```python
from build123d import *

# Parameters (mm, degrees)
SKETCH1_R                   = 3
BOSS_EXTRUDE1_DEPTH         = 36
TAP_DRILL_FOR_M3_TAP1_D     = 2.5
TAP_DRILL_FOR_M3_TAP1_DEPTH = 10
TAP_DRILL_FOR_M3_TAP1_TIP   = 0.751075774
TAP_DRILL_FOR_M3_TAP2_D     = 2.5
TAP_DRILL_FOR_M3_TAP2_DEPTH = 10
TAP_DRILL_FOR_M3_TAP2_TIP   = 0.751075774


with BuildPart() as part:
    # Sketch1 → Boss-Extrude1 (new body)
    with BuildSketch(Plane(origin=(0, 0, 0), x_dir=(1, 0, 0), z_dir=(0, 1, 0))):
        Circle(SKETCH1_R)
    extrude(amount=BOSS_EXTRUDE1_DEPTH)

    # Tap Drill for M3 Tap1
    with Locations(Plane(origin=(0, 36, 0), x_dir=(1, 0, 0), z_dir=(0, 1, 0))):
        with Locations((0, 0)):
            Hole(TAP_DRILL_FOR_M3_TAP1_D / 2, depth=TAP_DRILL_FOR_M3_TAP1_DEPTH)
            with Locations((0, 0, -(TAP_DRILL_FOR_M3_TAP1_DEPTH + TAP_DRILL_FOR_M3_TAP1_TIP / 2))):  # 118° drill point
                Cone(0, TAP_DRILL_FOR_M3_TAP1_D / 2, TAP_DRILL_FOR_M3_TAP1_TIP, mode=Mode.SUBTRACT)

    # Tap Drill for M3 Tap2
    with Locations(Plane(origin=(0, 0, 0), x_dir=(-1, 0, 0), z_dir=(0, -1, 0))):
        with Locations((0, 0)):
            Hole(TAP_DRILL_FOR_M3_TAP2_D / 2, depth=TAP_DRILL_FOR_M3_TAP2_DEPTH)
            with Locations((0, 0, -(TAP_DRILL_FOR_M3_TAP2_DEPTH + TAP_DRILL_FOR_M3_TAP2_TIP / 2))):  # 118° drill point
                Cone(0, TAP_DRILL_FOR_M3_TAP2_D / 2, TAP_DRILL_FOR_M3_TAP2_TIP, mode=Mode.SUBTRACT)


solid = part.part
```
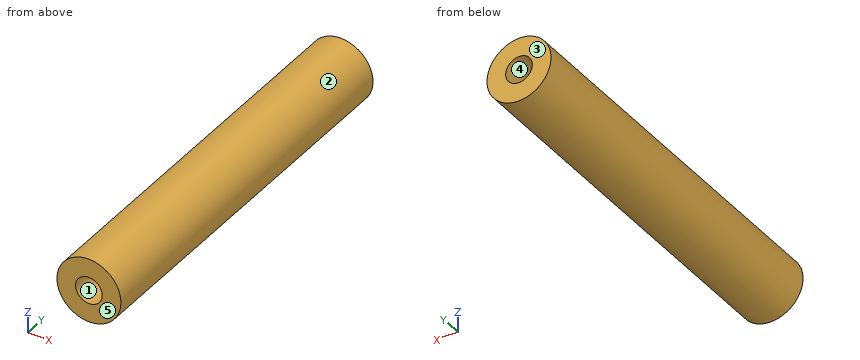
Design review of the part built by this model. Coordinates are the model's own, in mm. Face numbers are marked on the shaded views. A direction names the side the tool comes from. Round coordinates to 2 decimals unless told otherwise and drop trailing zeros. Write each loop counter-clockwise with the first axis right and the second up, starting at its lowest first coordinate (ties: lowest second). Pieces come first, ordered by that corner, then holes. Notation, with made-up numbers: (56, 67) -> (82, 67) arc R8 cw to (82, 73) -> close; hole circle Ø8 at (3.25, 75.25). An arc over 180 degrees is marked (long way). Answer in a Markdown table with one row per item.
Q1. Draft analysis for pull direction Z (two halves, no side actions). For the marked faces 1, 2 and 3, state which applies: +Z half, -Z half, draft (parallel to the pull), parting line (faces both ways), or undercut.
The answers:
| item | result |
|---|---|
| face 1 | undercut |
| face 2 | parting line |
| face 3 | draft |
Q2. Take a section at B-B, the plane z = -2.5. State the section outline as (x, y) points, then the cut area to 3 significant figures.
The answers:
| item | result |
|---|---|
| outline | (-1.66, 0) -> (1.66, 0) -> (1.66, 36) -> (-1.66, 36) -> close |
| area | 119 mm² |
Q3. Take a section at D-D, the plane x = 2.25. State the section outline as (y, z) points, then the cut area to 3 significant figures.
The answers:
| item | result |
|---|---|
| outline | (0, -1.98) -> (36, -1.98) -> (36, 1.98) -> (0, 1.98) -> close |
| area | 143 mm² |
Q4. Take a section at C-C, the plane y = 18. State the section outline as (x, z) points, then the cut area to 3 significant figures.
The answers:
| item | result |
|---|---|
| outline | circle Ø6 at (0, 0) |
| area | 28.3 mm² |
Q5. For the marked faces 4 and 5, list the 3-axis set-ups (+Z, -Z, +X, -X, +Y, -Y) from which the entire face can be reached by the end or side of a thin tool; tool diameter is ignored.
The answers:
| item | result |
|---|---|
| face 4 | +Y |
| face 5 | +Z, -Z, +X, -X, -Y |
Q6. Clearance check with flat-ended pins moving along their axes: pin 1 Ø3 at (y, z) = (9, -0.5) entering from +X; pin 2 Ø2 at (x, z) = (0, 0) entering from -Y; pin 3 Ø1.5 at (x, y) = (-2, 22.5) entering from +Z; pin 4 Ø1.5 at (x, z) = (0, 0) entering from -Y. State where each tip first meets the part, or that it passes through.
The answers:
| item | result |
|---|---|
| pin 1 | x = 3 |
| pin 2 | y = 10.15 |
| pin 3 | z = 2.73 |
| pin 4 | y = 10.3 |
Q7. Take a section at A-A, the plane y = 8. State the section outline as (x, z) points.
The answers:
| item | result |
|---|---|
| outline | circle Ø6 at (0, 0); hole circle Ø2.5 at (0, 0) |
Q8. To check wall thickness, follow L1, parallel to Z at x = 0, y = 3.5; L2, parallel to Z at x = 0.2, y = 25; L3, parallel to Z at x = -0.9, y = 6.5. State the ranges of each line that lie inside material, in increasing order. Write a range as [from, to].
The answers:
| item | result |
|---|---|
| L1 | [-3, -1.25], [1.25, 3] |
| L2 | [-2.99, 2.99] |
| L3 | [-2.86, -0.87], [0.87, 2.86] |
